from build123d import *

# Parameters (mm, degrees)
SKETCH1_R           = 40
SKETCH1_R_2         = 4.1
SKETCH1_R_3         = 1
SKETCH1_R_4         = 2.5
BOSS_EXTRUDE1_DEPTH = 3.175


with BuildPart() as part:
    # Sketch1 → Boss-Extrude1 (new body)
    with BuildSketch(Plane.XY):
        Circle(SKETCH1_R)
        Circle(SKETCH1_R_2, mode=Mode.SUBTRACT)
        with Locations((10, 0)):
            Circle(SKETCH1_R_3, mode=Mode.SUBTRACT)
        with Locations((0, -10)):
            Circle(SKETCH1_R_3, mode=Mode.SUBTRACT)
        with Locations((-10, 0)):
            Circle(SKETCH1_R_3, mode=Mode.SUBTRACT)
        with Locations((0, 10)):
            Circle(SKETCH1_R_3, mode=Mode.SUBTRACT)
        with Locations((0, 32.500000024)):
            Circle(SKETCH1_R_4, mode=Mode.SUBTRACT)
        with Locations((32.500000024, 0)):
            Circle(SKETCH1_R_4, mode=Mode.SUBTRACT)
        with Locations((0, -32.500000024)):
            Circle(SKETCH1_R_4, mode=Mode.SUBTRACT)
        with Locations((-32.500000024, 0)):
            Circle(SKETCH1_R_4, mode=Mode.SUBTRACT)
        with BuildLine():
            ThreePointArc((1.5, 16.564017782), (17.18320836, 14.289419004), (31.574025173, 7.653063411))
            ThreePointArc((31.574025173, 7.653063411), (32.247204442, 5.433888763), (29.939339852, 5.206583941))
            ThreePointArc((29.939339852, 5.206583941), (16.320954352, 11.431399277), (1.5, 13.564017782))
            ThreePointArc((1.5, 13.564017782), (0, 15.064017782), (1.5, 16.564017782))
        make_face(mode=Mode.SUBTRACT)
        with BuildLine():
            ThreePointArc((16.564017782, -1.5), (14.289419004, -17.18320836), (7.653063411, -31.574025173))
            ThreePointArc((7.653063411, -31.574025173), (5.433888763, -32.247204442), (5.206583941, -29.939339852))
            ThreePointArc((5.206583941, -29.939339852), (11.431399277, -16.320954352), (13.564017782, -1.5))
            ThreePointArc((13.564017782, -1.5), (15.064017782, 0), (16.564017782, -1.5))
        make_face(mode=Mode.SUBTRACT)
        with BuildLine():
            ThreePointArc((-1.5, -16.564017782), (-17.18320836, -14.289419004), (-31.574025173, -7.653063411))
            ThreePointArc((-31.574025173, -7.653063411), (-32.247204442, -5.433888763), (-29.939339852, -5.206583941))
            ThreePointArc((-29.939339852, -5.206583941), (-16.320954352, -11.431399277), (-1.5, -13.564017782))
            ThreePointArc((-1.5, -13.564017782), (0, -15.064017782), (-1.5, -16.564017782))
        make_face(mode=Mode.SUBTRACT)
        with BuildLine():
            ThreePointArc((-16.564017782, 1.5), (-14.289419004, 17.18320836), (-7.653063411, 31.574025173))
            ThreePointArc((-7.653063411, 31.574025173), (-5.433888763, 32.247204442), (-5.206583941, 29.939339852))
            ThreePointArc((-5.206583941, 29.939339852), (-11.431399277, 16.320954352), (-13.564017782, 1.5))
            ThreePointArc((-13.564017782, 1.5), (-15.064017782, 0), (-16.564017782, 1.5))
        make_face(mode=Mode.SUBTRACT)
    extrude(amount=BOSS_EXTRUDE1_DEPTH)


solid = part.part
For this review, take the finished solid that the model builds, in its own axes (mm). Round coordinates to 2 decimals unless told otherwise and drop trailing zeros. Write each loop counter-clockwise with the first axis right and the second up, starting at its lowest first coordinate (ties: lowest second). Pieces come first, ordered by that corner, then holes. Notation, with made-up numbers: M 49.25,-25 L 65.25,-25 A18 cw 65.25,0 Z; hole C -33.75,20 d10. An arc over 180 degrees is marked long. Write item = value, one per line. Start each with the question number.
(1) We need section A-A (y = 12). Give the boundary of the cut face in (x, z) (3 decimals), then the cut area to 3 significant figures.
(2) The part is to be moulded in two halves that separate along X. For faces 1 (the face through (-8.67, -39.05, 1.57)), 2 (the face through (-1, -8, 3.175)), 3 (the face through (11.372, -16.523, 1.565)), say which applies: +X half, -X half, draft (parallel to the pull), parting line (faces both ways), or undercut.
(3) We need section C-C (z = 2.5). Give the number of separate pieces and of enclosed holes in the cut face, then the cut area to 3 significant figures.
(4) Clearance check with flat-ended pins moving along their axes: pin 1 Ø3 at (x, y) = (32.5, 0) entering from +Z; pin 2 Ø1.5 at (y, z) = (-18.5, 0.5) entering from -X. State where each tip first meets the part, or that it passes through.
(5) We need section B-B (x = -15.5). Give the boundary of the cut face in (y, z) (3 decimals), then the cut area to 3 significant figures.
(6) For line 1 along X through (y, z) = (-31, 0.95); line 2 along Y through (x, z) = (6, 2.9); line 3 along X through (y, z) = (-7, 1.6), list the stretches that pass through material, from the lowest coordinate up.
(7) We need section D-D (x = 34). Give the boundary of the cut face in (y, z) (3 decimals), then the cut area to 3 significant figures.
Results found:
q1.outline = M -38.158,0 L -15.556,0 L -15.556,3.175 L -38.158,3.175 Z; M -12.505,0 L 14.227,0 L 14.227,3.175 L -12.505,3.175 Z; M 23.479,0 L 38.158,0 L 38.158,3.175 L 23.479,3.175 Z
q1.area = 203 mm²
q2.face_1 = parting line
q2.face_2 = draft
q2.face_3 = undercut
q3.separate_pieces = 1
q3.enclosed_holes = 13
q3.area = 4,480 mm²
q4.pin_1 = through
q4.pin_2 = -35.85
q5.outline = M -36.875,0 L -14.759,0 L -14.759,3.175 L -36.875,3.175 Z; M -11.665,0 L 0.065,0 L 0.065,3.175 L -11.665,3.175 Z; M 12.286,0 L 36.875,0 L 36.875,3.175 L 12.286,3.175 Z
q5.area = 186 mm²
q6.line_1 = -25.28 to -2, 2 to 4.77, 8.02 to 25.28
q6.line_2 = -39.55 to -32.48, -28.67 to 13.37, 16.38 to 39.55
q6.line_3 = -39.38 to -32.31, -26.94 to 13.28, 16.29 to 39.38
q7.outline = M -21.071,0 L -2,0 L -2,3.175 L -21.071,3.175 Z; M 2,0 L 21.071,0 L 21.071,3.175 L 2,3.175 Z
q7.area = 121 mm²
